Verification items for the finished model (mm, model axes). Face numbers are marked on the shaded views. A direction names the side the tool comes from. Coordinates: 2 decimals unless noted, no trailing zeros. Loops run counter-clockwise (first coordinate to the right, second up) from the corner with the lowest first, then second, coordinate; pieces in that order, holes last.
Q1. Mould release check, pull along Y, two halves, no side actions. Record for the marked faces 4, 5 and 6: +Y half, -Y half, draft (parallel to the pull), parting line (faces both ways), or undercut.
Q2. Access from +Z, -Z, +X, -X, +Y, -Y to the whole of each face (thin tool, end or side, straight path). Record for the marked faces 1, 2 and 3.
Q3. Sectioned sample at D-D (y = 12). Enter the section's corners in (x, z), then the cut area to 3 significant figures.
Q4. Sectioned sample at B-B (x = 0). Enter the section's corners in (y, z).
Q5. Sectioned sample at A-A (y = 0). Enter the section's corners in (x, z), then the cut area to 4 significant figures.
Q6. Material ranges on probe 1 along X at (y, z) = (11.75, 17); probe 2 along X at (y, z) = (-7.25, 18); probe 3 along X at (y, z) = (-0.75, 24.5), recorded low to high.
Q7. Sectioned sample at C-C (z = -3). Enter the section's corners in (x, y), then the cut area to 3 significant figures.
Q8. Go/stop test with flat-tipped pins: P1, Ø1.5, axis at y = -5.5, z = 3, coming from the +X side; P2, Ø3, axis at y = 11, z = 14.5, coming from the +X side; P3, Ø3, axis at x = 6.5, z = 0.5, coming from the +Y side; P4, Ø7, axis at x = 0, y = 0, coming from the -Z side. Record where each tip stops, or that it passes through.
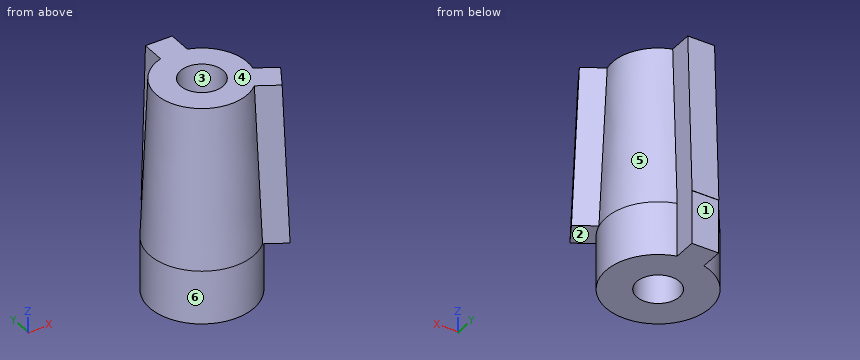
```python
from build123d import *

# Parameters (mm, degrees)
SKETCH1_R           = 8.5
SKETCH1_R_2         = 4
BOSS_EXTRUDE1_DEPTH = 30
SKETCH2_R           = 9.75
BOSS_EXTRUDE2_DEPTH = 10
SKETCH4_R           = 4
CUT_EXTRUDE1_DEPTH  = 40
SKETCH6_W           = 5
SKETCH6_H           = 6.142281657
SKETCH5_W           = 5
SKETCH5_H           = 5.134988922
CIRPATTERN1_COUNT   = 2
CIRPATTERN1_ANGLE   = 240
SKETCH7_W           = 5
SKETCH7_H           = 5.55011225
BOSS_EXTRUDE3_DEPTH = 10


with BuildPart() as part:
    # Sketch1 → Boss-Extrude1 (new body)
    with BuildSketch(Plane.XY):
        Circle(SKETCH1_R)
        Circle(SKETCH1_R_2, mode=Mode.SUBTRACT)
    extrude(amount=BOSS_EXTRUDE1_DEPTH)

    # Sketch2 → Boss-Extrude2 (add)
    with BuildSketch(Plane(origin=(0, 0, 0), x_dir=(-1, 0, 0), z_dir=(0, 0, -1))):
        Circle(SKETCH2_R)
    extrude(amount=BOSS_EXTRUDE2_DEPTH)

    # loft up to a face of the part (loft4)
    loft([Face(Wire([part.edges().sort_by_distance((-5.8186504, 6.196233333, 30))[0]])), Face(Wire([part.edges().sort_by_distance((6.674334283, -7.107444117, 0))[0]]))])

    # Sketch4 → Cut-Extrude1 (cut)
    with BuildSketch(Plane.XY.offset(30)):
        Circle(SKETCH4_R)
    extrude(amount=-CUT_EXTRUDE1_DEPTH, mode=Mode.SUBTRACT)

    # Sketch6 → Loft5 section 0
    with BuildSketch(Plane.XY.offset(30)):
        with Locations((0, 9.428859172)):
            Rectangle(SKETCH6_W, SKETCH6_H)
    # Sketch5 → Loft5 section 1
    with BuildSketch(Plane.XY):
        with Locations((0, 11.182505539)):
            Rectangle(SKETCH5_W, SKETCH5_H)
    loft5 = loft()

    # CirPattern1: Loft5 ×2 about axis
    cirpattern1_axis = Axis((0, 0, 0), (0, 0, 1))
    for i in range(1, CIRPATTERN1_COUNT):
        add(loft5.rotate(cirpattern1_axis, i * CIRPATTERN1_ANGLE / (CIRPATTERN1_COUNT - 1)))

    # Sketch7 → Boss-Extrude3 (add)
    with BuildSketch(Plane(origin=(0, 0, -10), x_dir=(-1, 0, 0), z_dir=(0, 0, -1))):
        with Locations((0, 10.919421432)):
            Rectangle(SKETCH7_W, SKETCH7_H)
    extrude(amount=-BOSS_EXTRUDE3_DEPTH)


solid = part.part
```
Geometry check:
1. face 4: draft
1. face 5: undercut
1. face 6: parting line
2. face 1: -Z, +X, -X, +Y
2. face 2: -Z, +X, -Y
2. face 3: +Z, -Z
3. outline: (-2.5, -10) - (2.5, -10) - (2.5, 30) - (-2.5, 30) - close
3. area: 200 mm2
4. outline: (-9.75, -10) - (-4, -10) - (-4, 30) - (-8.5, 30) - (-9.75, 0) - close; (4, -10) - (13.69, -10) - (13.69, 0) - (13.75, 0) - (12.5, 30) - (4, 30) - close
5. outline: (-9.75, -10) - (-4, -10) - (-4, 30) - (-8.5, 30) - (-9.75, 0) - close; (4, -10) - (9.75, -10) - (9.75, 0) - (8.5, 30) - (4, 30) - close
5. area: 422.5 mm2
6. probe 1: x = -2.5 to 2.5
6. probe 2: x = -5.33 to 5.33, 7.56 to 10.83
6. probe 3: x = -8.7 to -3.93, 3.93 to 8.7
7. outline: (-2.5, 9.42) arc R9.75 ccw (long way) to (2.5, 9.42) - (2.5, 13.69) - (-2.5, 13.69) - close; hole circle Ø8 at (0, 0)
7. area: 269 mm2
8. P1: stops at x = 12.99
8. P2: stops at x = 2.5
8. P3: stops at y = 8.35
8. P4: passes through
